Read the model definition and answer for the solid it produces. Units are mm, in the model's axes. A direction names the side the tool comes from. Round coordinates to 2 decimals unless told otherwise and drop trailing zeros. Order: outer loops, then holes, each group sorted by start corner. A loop starts at its lowest first (then second) coordinate and runs counter-clockwise, first axis right, second up. Notation, with made-up numbers: M 30.5,-29 L 42.5,-29 A14 ccw 42.5,-4 Z; hole C -17.5,-2 d2. An arc over 180 degrees is marked long. Answer as CSV lines item,"result".
```python
from build123d import *

# Parameters (mm, degrees)
F1_DEPTH = 1260
F2_W     = 1220
F2_H     = 490
F2_W_2   = 1160
F2_H_2   = 430
F3_DEPTH = 30
F4_W     = 30
F4_H     = 490
F5_DEPTH = 210


with BuildPart() as f1:
    # F0 (on Right) → F1 (new body)
    with BuildSketch(Plane.YZ):
        Polygon((-680, 0), (-150, 0), (0, 800), (-38.217112, 799.071343), (-38.217112, 820), (0, 820), (0, 1000), (-130, 1000), (-130, 820), (-71.854167, 820), (-71.854167, 798.25398), (-153.312458, 796.274585), (-274.488943, 150), (-680, 150), align=None)
    extrude(amount=F1_DEPTH)

    # F2 (on face) → F3 (join)
    with BuildSketch(Plane(origin=(0, 0, 0), x_dir=(1, 0, 0), z_dir=(0, 0, -1))):
        with Locations((630, 415)):
            Rectangle(F2_W, F2_H)
        with Locations((630, 415)):
            Rectangle(F2_W_2, F2_H_2, mode=Mode.SUBTRACT)
    extrude(amount=F3_DEPTH)

    # F4 (on face) → F5 (join)
    with BuildSketch(Plane(origin=(0, 0, -30), x_dir=(1, 0, 0), z_dir=(0, 0, -1))):
        with Locations((1090.837493, 415)):
            Rectangle(F4_W, F4_H)
        with Locations((637.32095, 415)):
            Rectangle(F4_W, F4_H)
        with Locations((90.456768, 415)):
            Rectangle(F4_W, F4_H)
    extrude(amount=F5_DEPTH)


solid = f1.part
```
Item 1: A cutting plane is placed at D-D, the plane y = -257. Determine the outline of the cut face in (x, z), and give its area (3 significant figures).
Ans:
outline,"M 0,0 L 20,0 L 20,-30 L 50,-30 L 50,0 L 1210,0 L 1210,-30 L 1240,-30 L 1240,0 L 1260,0 L 1260,243.27 L 0,243.27 Z; M 75.46,-240 L 105.46,-240 L 105.46,-30 L 75.46,-30 Z; M 622.32,-240 L 652.32,-240 L 652.32,-30 L 622.32,-30 Z; M 1075.84,-240 L 1105.84,-240 L 1105.84,-30 L 1075.84,-30 Z"
area,"327,000 mm2"
Item 2: A cutting plane is placed at B-B, the plane y = -505.5. Determine the outline of the cut face in (x, z).
Ans:
outline,"M 0,0 L 20,0 L 20,-30 L 50,-30 L 50,0 L 1210,0 L 1210,-30 L 1240,-30 L 1240,0 L 1260,0 L 1260,150 L 0,150 Z; M 75.46,-240 L 105.46,-240 L 105.46,-30 L 75.46,-30 Z; M 622.32,-240 L 652.32,-240 L 652.32,-30 L 622.32,-30 Z; M 1075.84,-240 L 1105.84,-240 L 1105.84,-30 L 1075.84,-30 Z"
Item 3: Determine the mould class of faces 1 (the face through (360, -185, -30)), 2 (the face through (1222, -416, -30)), 3 (the face through (1240, -412, -15)), 4 (the face through (1091, -418, -30)) for opening direction X: +X half, -X half, draft (parallel to the pull), parting line (faces both ways), or undercut.
Ans:
face 1,"undercut"
face 2,"draft"
face 3,"+X half"
face 4,"undercut"
Item 4: A cutting plane is placed at A-A, the plane z = -51. Determine the outline of the cut face in (x, y), and give its area (3 significant figures).
Ans:
outline,"M 75.46,-660 L 105.46,-660 L 105.46,-170 L 75.46,-170 Z; M 622.32,-660 L 652.32,-660 L 652.32,-170 L 622.32,-170 Z; M 1075.84,-660 L 1105.84,-660 L 1105.84,-170 L 1075.84,-170 Z"
area,"44,100 mm2"
Item 5: Find the intervals of material crossed by probe 1 along X at (y, z) = (-508, -171.5); probe 2 along Z at (x, y) = (1133, -589.5); probe 3 along Y at (x, z) = (777.5, 894), in increasing order. Write a range as [from, to].
Ans:
probe 1,"[75.46, 105.46], [622.32, 652.32], [1075.84, 1105.84]"
probe 2,"[0, 150]"
probe 3,"[-130, 0]"
Item 6: A cutting plane is placed at C-C, the plane x = 681. Determine the outline of the cut face in (y, z), and give its area (3 significant figures).
Ans:
outline,"M -680,0 L -660,0 L -660,-30 L -630,-30 L -630,0 L -200,0 L -200,-30 L -170,-30 L -170,0 L -150,0 L 0,800 L -38.22,799.07 L -38.22,820 L 0,820 L 0,1000 L -130,1000 L -130,820 L -71.85,820 L -71.85,798.25 L -153.31,796.27 L -274.49,150 L -680,150 Z"
area,"206,000 mm2"
Item 7: Flat-ended cylindrical pins translate along their axes: pin 1 (8 mm diameter, centred on x = 274.5, y = -547.5, fed in from +Z); pin 2 (1.5 mm diameter, centred on x = 542.5, z = 232, fed in from +Y); pin 3 (1.5 mm diameter, centred on x = 577, z = 875, fed in from -Y). Find the tip coordinate at first contact, or state that the pin passes through.
Ans:
pin 1,"z = 150"
pin 2,"y = -106.36"
pin 3,"y = -130"
Item 8: A tool of negligible diameter and unlimited length cuts with its end or side. For faces 5 (the face through (1075.837, -412, -134)), 6 (the face through (621, -19, 820)), 7 (the face through (20, -412, -15)), from which of +Z, -Z, +X, -X, +Y, -Y can it reach the whole face along a straight path? Write none if from no direction.
Ans:
face 5,"-Z, +Y, -Y"
face 6,"+X, -X, +Y"
face 7,"-Z, -X, +Y, -Y"
